```python
from build123d import *

# Parameters (mm, degrees)
SKETCH1_W                    = 21
SKETCH1_H                    = 50
BASE_FLANGE1_DEPTH           = 3
HEM1_START                   = -25
HEM1_DEPTH                   = 12.5
LPATTERN1_COUNT              = 2
LPATTERN1_PITCH              = 25
SKETCH9_W                    = 5.5
SKETCH9_H                    = 12.5
CUT_EXTRUDE5_DEPTH           = 3
F_6_0_6_DIAMETER_HOLE1_D     = 6
F_6_0_6_DIAMETER_HOLE1_DEPTH = 8
F_6_0_6_DIAMETER_HOLE1_TIP   = 1.802581857
CHAMFER1_SIZE                = 0.5


# Read off the part's stored shape, not the designer's step: Hem1
# Sheet-metal steps are written as plain solids
with BuildPart() as part:
    # Sketch1 → Base-Flange1 (new body)
    with BuildSketch(Plane.XY):
        Rectangle(SKETCH1_W, SKETCH1_H)
    extrude(amount=BASE_FLANGE1_DEPTH)

    # Hem1 outline → Hem1 (add)
    with BuildSketch(Plane(origin=(0, 0, 0), x_dir=(1, 0, 0), z_dir=(0, 1, 0)).offset(HEM1_START)):
        with BuildLine():
            Line((8.150768448, -4.644949642), (5.331690586, -3.618889212))
            ThreePointArc((5.331690586, -3.618889212), (13.654670401, -10.005336243), (10.5, 0))
            Line((10.5, 0), (10.5, -3))
            ThreePointArc((10.5, -3), (11.933941091, -7.547880111), (8.150768448, -4.644949642))
        make_face()
    hem1 = extrude(amount=HEM1_DEPTH)

    # LPattern1: Hem1 ×2
    with Locations(*[(0, i * LPATTERN1_PITCH, 0) for i in range(1, LPATTERN1_COUNT)]):
        add(hem1)

    # Sketch9 → Cut-Extrude5 (cut)
    with BuildSketch(Plane.XY.offset(3)):
        with Locations((7.75, 18.75)):
            Rectangle(SKETCH9_W, SKETCH9_H)
        with Locations((7.75, -6.25)):
            Rectangle(SKETCH9_W, SKETCH9_H)
    extrude(amount=-CUT_EXTRUDE5_DEPTH, mode=Mode.SUBTRACT)

    # Ø6.0 (6) Diameter Hole1
    with Locations(Plane(origin=(-2.5, 15, 3), x_dir=(1, 0, 0), z_dir=(0, 0, 1))):
        with Locations((0, 0), (0, -30)):
            Hole(F_6_0_6_DIAMETER_HOLE1_D / 2, depth=F_6_0_6_DIAMETER_HOLE1_DEPTH)
            with Locations((0, 0, -(F_6_0_6_DIAMETER_HOLE1_DEPTH + F_6_0_6_DIAMETER_HOLE1_TIP / 2))):  # 118° drill point
                Cone(0, F_6_0_6_DIAMETER_HOLE1_D / 2, F_6_0_6_DIAMETER_HOLE1_TIP, mode=Mode.SUBTRACT)

    # Chamfer1
    chamfer1_edges = [part.edges().sort_by_distance(p)[0] for p in [
        (-10.5, 0, 3),
        (0.5, -15, 3),
        (0.5, 15, 3),
    ]]
    chamfer(chamfer1_edges, length=CHAMFER1_SIZE)


solid = part.part
```
Work out the finished part from the listing and answer in its coordinate system (mm). A direction names the side the tool comes from. Give positions to 0.01 mm unless a question says otherwise; leave off trailing zeros. Order: outer loops, then holes, each group sorted by start corner. A loop starts at its lowest first (then second) coordinate and runs counter-clockwise, first axis right, second up.
1. Section C-C, the plane x = -2.5 is taken. Determine the outline of the cut face in (y, z), and give its area (4 significant figures).
Result sheet:
outline: (-25, 0) - (-18, 0) - (-18, 2.5) - (-18.5, 3) - (-25, 3) - close; (-12, 0) - (12, 0) - (12, 2.5) - (11.5, 3) - (-11.5, 3) - (-12, 2.5) - close; (18, 0) - (25, 0) - (25, 3) - (18.5, 3) - (18, 2.5) - close
area: 113.5 mm2
2. Section D-D, the plane y = 1.5 is taken. Determine the outline of the cut face in (x, z).
Result sheet:
outline: (-10.5, 0) - (10.5, 0) arc R5.5 ccw (long way) to (5.33, 3.62) - (8.15, 4.64) arc R2.5 cw (long way) to (10.5, 3) - (-10, 3) - (-10.5, 2.5) - close
3. Section B-B, the plane y = -15 is taken. Determine the outline of the cut face in (x, z), and give its area (3 significant figures).
Result sheet:
outline: (-10.5, 0) - (-5.5, 0) - (-5.5, 2.5) - (-6, 3) - (-10, 3) - (-10.5, 2.5) - close; (0.5, 0) - (10.5, 0) arc R5.5 ccw (long way) to (5.33, 3.62) - (8.15, 4.64) arc R2.5 cw (long way) to (10.5, 3) - (1, 3) - (0.5, 2.5) - close
area: 105 mm2
4. Section A-A, the plane z = 5.5 is taken. Determine the outline of the cut face in (x, y).
Result sheet:
outline: (5, -25) - (8, -25) - (8, -12.5) - (5, -12.5) - close; (5, 0) - (8, 0) - (8, 12.5) - (5, 12.5) - close; (13, -25) - (16, -25) - (16, -12.5) - (13, -12.5) - close; (13, 0) - (16, 0) - (16, 12.5) - (13, 12.5) - close
5. Each of these flat-tipped pins is pushed along its axis until it touches: P1, Ø0.9, axis at y = 20.5, z = 1.5, coming from the +X side; P2, Ø1, axis at y = 3.5, z = 7.5, coming from the +X side; P3, Ø4, axis at y = 2.5, z = 9, coming from the -X side. Where does it stop, or does it pass through?
Result sheet:
P1: stops at x = 5
P2: stops at x = 15.79
P3: stops at x = 5.21
6. For faces 1 (the flat face through (6.76, 6.16, 4.14)), 2 (the flat face through (0, 0, 3)), 3 (the flat face through (5, 19, 2)), 4 (the flat face through (5, -6, 2)), determine the directions among +Z, -Z, +X, -X, +Y, -Y from which every point of the face is accessible in a straight line to the end or side of a thin tool.
Result sheet:
face 1: +Y, -Y
face 2: -X, +Y, -Y
face 3: +Z, -Z, +X, +Y
face 4: +Z, -Z, +X
7. The mould has two halves that part along Y. Classify faces 5 (the flat face through (12, 12.5, 3)), 6 (the cylindrical face through (13.493, 6.163, 10.114)), 7 (the cylindrical face through (-1.85, -17.93, 1.23)): released by +Y, released by -Y, zero draft, split by the parting line, or undercut.
Result sheet:
face 5: released by +Y
face 6: zero draft
face 7: undercut
8. Straight lines are drawn through the part: L1, parallel to Y at x = -2.5, z = 1.2; L2, parallel to Y at x = 9.5, z = 2.25; L3, parallel to Z at x = 10.5, y = 8.75. For each, find the intervals that lie inside material, in ascending order.
Result sheet:
L1: y = -25 to -18, -12 to 12, 18 to 25
L2: y = -25 to -12.5, 0 to 12.5
L3: z = 0 to 3, 8 to 11
